Geometry: final body of the model. Coordinates: model frame, mm. Face numbers are marked on the shaded views. Round coordinates to 2 decimals unless told otherwise and drop trailing zeros. Loops run counter-clockwise (first coordinate to the right, second up) from the corner with the lowest first, then second, coordinate; pieces in that order, holes last. Notation, with made-up numbers: (46.5, 48) - (78.5, 48) arc R21 ccw to (78.5, 82) - close; hole circle Ø11 at (81, 79). An arc over 180 degrees is marked (long way). Use CSV: the item, a comma, the result in double quotes.
from build123d import *

# Parameters (mm, degrees)
EXTRUDE_1_DEPTH              = 30
HOLE_WIZARD_M3_2_D           = 3.4
HOLE_WIZARD_M3_2_ON_FACE_2_D = 3.4


with BuildPart() as part:
    # 스케치1 → 보스-돌출1 (new body)
    with BuildSketch(Plane.XY):
        Polygon((1.443375673, -2.5), (2.886751346, 0), (1.443375673, 2.5), (-1.443375673, 2.5), (-2.886751346, 0), (-1.443375673, -2.5), align=None)
    extrude(amount=EXTRUDE_1_DEPTH)

    # M3 여유 구멍2 (through all)
    with Locations(Plane(origin=(0, 0, 0), x_dir=(-1, 0, 0), z_dir=(0, 0, -1))):
        with Locations((0, 0)):
            Hole(HOLE_WIZARD_M3_2_D / 2)

    # M3 여유 구멍2 on face 2 (through all)
    with Locations(Plane.XY.offset(30)):
        with Locations((0, 0)):
            Hole(HOLE_WIZARD_M3_2_ON_FACE_2_D / 2)


solid = part.part
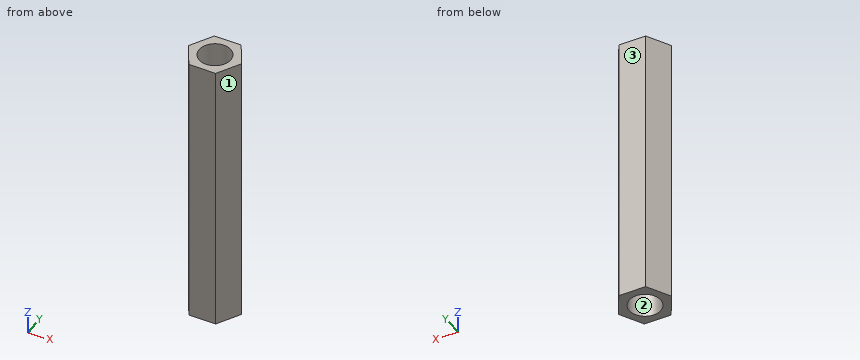
Item 1: Section A-A on z = 6.5. Return the cut outline in (x, y).
Final values:
outline,"(-2.89, 0) - (-1.44, -2.5) - (1.44, -2.5) - (2.89, 0) - (1.44, 2.5) - (-1.44, 2.5) - close; hole circle Ø3.4 at (0, 0)"
Item 2: Pin query (flat end, axial travel): P1, Ø2, axis at y = 2, z = 9.5, coming from the +X side. Return the tip coordinate at first contact, or that it passes through.
Final values:
P1,"stops at x = 2.31"
Item 3: Material intervals for line 1 (Y direction, x = 0, z = 7); line 2 (Y direction, x = 1.55, z = 4.5); line 3 (X direction, y = 0.35, z = 5.5), sorted ascending.
Final values:
line 1,"y = -2.5 to -1.7, 1.7 to 2.5"
line 2,"y = -2.32 to -0.7, 0.7 to 2.32"
line 3,"x = -2.68 to -1.66, 1.66 to 2.68"
Item 4: Mould query, pull axis Y, two halves, no side actions, for the marked faces 1, 2 and 3. Classes: released by +Y, released by -Y, zero draft, split by the parting line, or undercut.
Final values:
face 1,"released by -Y"
face 2,"undercut"
face 3,"released by +Y"
Item 5: Section D-D on y = -2.15. Return the cut outline in (x, z), plus the area to 3 significant figures.
Final values:
outline,"(-1.65, 0) - (1.65, 0) - (1.65, 30) - (-1.65, 30) - close"
area,"98.7 mm²"
Item 6: Section C-C on y = 0.75. Return the cut outline in (x, z).
Final values:
outline,"(-2.45, 0) - (-1.53, 0) - (-1.53, 30) - (-2.45, 30) - close; (1.53, 0) - (2.45, 0) - (2.45, 30) - (1.53, 30) - close"
Item 7: Section B-B on x = 0. Return the cut outline in (y, z).
Final values:
outline,"(-2.5, 0) - (-1.7, 0) - (-1.7, 30) - (-2.5, 30) - close; (1.7, 0) - (2.5, 0) - (2.5, 30) - (1.7, 30) - close"
